The listing builds one solid part. Answer for the finished solid, in the listing's coordinates (mm). A direction names the side the tool comes from. Coordinates: 2 decimals unless noted, no trailing zeros. Loops run counter-clockwise (first coordinate to the right, second up) from the corner with the lowest first, then second, coordinate; pieces in that order, holes last. Notation, with made-up numbers: M -8,10 L 30,10 A9 cw 30,15 Z; hole C 40,-13.5 d1. An arc over 180 degrees is marked long. Answer as a JSON object with one key per item and string values. Group by question number.
1. For faces 1 (the face through (0, 3, 9)), 2 (the face through (0, 1, 20)), determine the directions among +Z, -Z, +X, -X, +Y, -Y from which every point of the face is accessible in a straight line to the end or side of a thin tool.
2. Straight lines are drawn through the part: L1, parallel to X at y = 8, z = -0.75; L2, parallel to X at y = 0.7, z = 10; L3, parallel to Y at x = -11, z = 14.75. For each, find the intervals that lie inside material, in ascending order.
3. A cutting plane is placed at A-A on x = 10. Give the vertices of the cut face in (y, z), and give its area (3 significant figures).
4. Given pin 1 (5 mm diameter, centred on x = 4, y = 18.5, fed in from +Z); pin 2 (5.5 mm diameter, centred on x = 10, z = 10, fed in from +Y), each flat-ended and moving along its own axis, determine where each tip first touches the part or whether it passes through.
5. A cutting plane is placed at C-C on z = 8.25. Give the vertices of the cut face in (x, y).
6. Determine the mould class of faces 3 (the face through (7.97, 1.52, 12.21)), 4 (the face through (-25, 9, 5)), 5 (the face through (0, 23, -4)) for opening direction X: released by +X, released by -X, zero draft, split by the parting line, or undercut.
7. A cutting plane is placed at D-D on y = 8.5. Give the vertices of the cut face in (x, z), and give its area (3 significant figures).
8. A cutting plane is placed at B-B on y = 1.5. Give the vertices of the cut face in (x, z).
from build123d import *

# Parameters (mm, degrees)
SKETCH_1_W          = 50
SKETCH_1_H          = 25.63
EXTRUDE_1_DEPTH     = 3
SKETCH_2_W          = 50
SKETCH_2_H          = 3
EXTRUDE_2_DEPTH     = 20
EXTRUDE_3_DEPTH     = 3
SKETCH_7_R          = 3
CUT_EXTRUDE_2_DEPTH = 38.749172176


with BuildPart() as part:
    # 草圖1 → 填料-伸長1 (new body)
    with BuildSketch(Plane(origin=(0, 0, 0), x_dir=(1, 0, 0), z_dir=(0, 1, 0))):
        with Locations((0, -7.185)):
            Rectangle(SKETCH_1_W, SKETCH_1_H)
    extrude(amount=EXTRUDE_1_DEPTH)

    # 草圖2 → 填料-伸長2 (add)
    with BuildSketch(Plane(origin=(0, 3, 0), x_dir=(1, 0, 0), z_dir=(0, 1, 0))):
        with Locations((0, 4.13)):
            Rectangle(SKETCH_2_W, SKETCH_2_H)
    extrude(amount=EXTRUDE_2_DEPTH)

    # 草圖6 → 填料-伸長3 (add)
    with BuildSketch(Plane.ZY.offset(25)):
        Polygon((-2.63, 23), (20, 3), (-2.63, 3), align=None)
    extrude_3 = extrude(amount=-EXTRUDE_3_DEPTH)

    # 鏡射1: 填料-伸長3 across plane
    add(extrude_3.mirror(Plane(origin=(0, 0, 0), x_dir=(0, 0, 1), z_dir=(1, 0, 0))))

    # 草圖7 → 除料-伸長2 (cut, through all)
    with BuildSketch(Plane(origin=(0, 3, 0), x_dir=(1, 0, 0), z_dir=(0, 1, 0))):
        with Locations(Location((-10, -10, 0), (0, 0, 270))):
            Circle(SKETCH_7_R)
        with Locations(Location((10, -10, 0), (0, 0, 90))):
            Circle(SKETCH_7_R)
    extrude(amount=-CUT_EXTRUDE_2_DEPTH, mode=Mode.SUBTRACT)


solid = part.part
From the geometry:
{
 "1": {"face 1": "+Z, +Y", "face 2": "+Z, +X, -X, +Y, -Y"},
 "2": {"L1": "x = -25 to -22, 22 to 25", "L2": "x = -25 to -13, -7 to 7, 13 to 25", "L3": "y = 0 to 3"},
 "3": {"outline": "M 0,-5.63 L 23,-5.63 L 23,-2.63 L 3,-2.63 L 3,7 L 0,7 Z; M 0,13 L 3,13 L 3,20 L 0,20 Z", "area": "119 mm²"},
 "4": {"pin 1": "stops at z = -2.63", "pin 2": "passes through"},
 "5": {"outline": "M -25,0 L -12.44,0 L -12.44,3 L -22,3 L -22,13.38 L -25,13.38 Z; M -7.56,0 L 7.56,0 L 7.56,3 L -7.56,3 Z; M 12.44,0 L 25,0 L 25,13.38 L 22,13.38 L 22,3 L 12.44,3 Z"},
 "6": {"face 3": "undercut", "face 4": "released by -X", "face 5": "zero draft"},
 "7": {"outline": "M -25,-5.63 L 25,-5.63 L 25,13.78 L 22,13.78 L 22,-2.63 L -22,-2.63 L -22,13.78 L -25,13.78 Z", "area": "248 mm²"},
 "8": {"outline": "M -25,-5.63 L 25,-5.63 L 25,20 L -25,20 Z; hole C -10,10 d6; hole C 10,10 d6"}
}
